from build123d import *

# Parameters (mm, degrees)
SKETCH1_R                  = 15
BOSS_EXTRUDE1_DEPTH        = 10
SKETCH2_R                  = 10.1
CUT_EXTRUDE1_DEPTH         = 20
SKETCH3_R                  = 15
BOSS_EXTRUDE2_DEPTH        = 10
SKETCH5_R                  = 10
CUT_EXTRUDE3_DEPTH         = 8
SKETCH8_W                  = 0.75
SKETCH8_H                  = 0.75
CUT_EXTRUDE5_DEPTH         = 2
FILL_START                 = -1.125
FILL_PATTERN2_OUTLINE_W    = 0.75
FILL_PATTERN2_OUTLINE_H    = 2
FILL_PATTERN2_DEPTH        = 0.75
FILL_START_2               = 0.375
FILL_PATTERN2_2_OUTLINE_W  = 0.75
FILL_PATTERN2_2_OUTLINE_H  = 2
FILL_PATTERN2_2_DEPTH      = 0.75
FILL_START_3               = -3.375
FILL_PATTERN2_3_OUTLINE_W  = 0.75
FILL_PATTERN2_3_OUTLINE_H  = 2
FILL_PATTERN2_3_DEPTH      = 0.75
FILL_START_4               = -1.875
FILL_PATTERN2_4_OUTLINE_W  = 0.75
FILL_PATTERN2_4_OUTLINE_H  = 2
FILL_PATTERN2_4_DEPTH      = 0.75
FILL_START_5               = 1.125
FILL_PATTERN2_5_OUTLINE_W  = 0.75
FILL_PATTERN2_5_OUTLINE_H  = 2
FILL_PATTERN2_5_DEPTH      = 0.75
FILL_START_6               = 2.625
FILL_PATTERN2_6_OUTLINE_W  = 0.75
FILL_PATTERN2_6_OUTLINE_H  = 2
FILL_PATTERN2_6_DEPTH      = 0.75
FILL_START_7               = -4.125
FILL_PATTERN2_7_OUTLINE_W  = 0.75
FILL_PATTERN2_7_OUTLINE_H  = 2
FILL_PATTERN2_7_DEPTH      = 0.75
FILL_START_8               = -2.625
FILL_PATTERN2_8_OUTLINE_W  = 0.75
FILL_PATTERN2_8_OUTLINE_H  = 2
FILL_PATTERN2_8_DEPTH      = 0.75
FILL_START_9               = -0.375
FILL_PATTERN2_9_OUTLINE_W  = 0.75
FILL_PATTERN2_9_OUTLINE_H  = 2
FILL_PATTERN2_9_DEPTH      = 0.75
FILL_START_10              = 1.875
FILL_PATTERN2_10_OUTLINE_W = 0.75
FILL_PATTERN2_10_OUTLINE_H = 2
FILL_PATTERN2_10_DEPTH     = 0.75
FILL_START_11              = 3.375
FILL_PATTERN2_11_OUTLINE_W = 0.75
FILL_PATTERN2_11_OUTLINE_H = 2
FILL_PATTERN2_11_DEPTH     = 0.75
SKETCH15_W                 = 16
SKETCH15_H                 = 2.5
SKETCH16_R                 = 1.2


# Read off the part's stored shape, not the designer's step: Fill Pattern2
with BuildPart() as part:
    # Sketch1 → Boss-Extrude1 (new body)
    with BuildSketch(Plane.XY):
        Circle(SKETCH1_R)
    extrude(amount=BOSS_EXTRUDE1_DEPTH)

    # Sketch2 → Cut-Extrude1 (cut)
    with BuildSketch(Plane.XY.offset(10)):
        Circle(SKETCH2_R)
    extrude(amount=-CUT_EXTRUDE1_DEPTH, mode=Mode.SUBTRACT)

    # Sketch3 → Boss-Extrude2 (add)
    with BuildSketch(Plane.XY.offset(10)):
        Circle(SKETCH3_R)
    extrude(amount=BOSS_EXTRUDE2_DEPTH)

    # Sketch5 → Cut-Extrude3 (cut)
    with BuildSketch(Plane.XY.offset(20)):
        Circle(SKETCH5_R)
    extrude(amount=-CUT_EXTRUDE3_DEPTH, mode=Mode.SUBTRACT)

    # Sketch8 → Cut-Extrude5 (cut)
    with BuildSketch(Plane(origin=(0, 0, 10), x_dir=(-1, 0, 0), z_dir=(0, 0, -1))):
        Rectangle(SKETCH8_W, SKETCH8_H)
    extrude(amount=-CUT_EXTRUDE5_DEPTH, mode=Mode.SUBTRACT)

    # Fill Pattern2 outline → Fill Pattern2 (cut)
    with BuildSketch(Plane.YZ.offset(FILL_START)):
        with Locations((-1.299038106, 11)):
            Rectangle(FILL_PATTERN2_OUTLINE_W, FILL_PATTERN2_OUTLINE_H)
        with Locations((1.299038106, 11)):
            Rectangle(FILL_PATTERN2_OUTLINE_W, FILL_PATTERN2_OUTLINE_H)
        with Locations((-3.897114317, 11)):
            Rectangle(FILL_PATTERN2_OUTLINE_W, FILL_PATTERN2_OUTLINE_H)
        with Locations((3.897114317, 11)):
            Rectangle(FILL_PATTERN2_OUTLINE_W, FILL_PATTERN2_OUTLINE_H)
    extrude(amount=FILL_PATTERN2_DEPTH, mode=Mode.SUBTRACT)

    # Fill Pattern2 2 outline → Fill Pattern2 2 (cut)
    with BuildSketch(Plane.YZ.offset(FILL_START_2)):
        with Locations((-1.299038106, 11)):
            Rectangle(FILL_PATTERN2_2_OUTLINE_W, FILL_PATTERN2_2_OUTLINE_H)
        with Locations((1.299038106, 11)):
            Rectangle(FILL_PATTERN2_2_OUTLINE_W, FILL_PATTERN2_2_OUTLINE_H)
        with Locations((-3.897114317, 11)):
            Rectangle(FILL_PATTERN2_2_OUTLINE_W, FILL_PATTERN2_2_OUTLINE_H)
        with Locations((3.897114317, 11)):
            Rectangle(FILL_PATTERN2_2_OUTLINE_W, FILL_PATTERN2_2_OUTLINE_H)
    extrude(amount=FILL_PATTERN2_2_DEPTH, mode=Mode.SUBTRACT)

    # Fill Pattern2 3 outline → Fill Pattern2 3 (cut)
    with BuildSketch(Plane.YZ.offset(FILL_START_3)):
        with Locations((0, 11)):
            Rectangle(FILL_PATTERN2_3_OUTLINE_W, FILL_PATTERN2_3_OUTLINE_H)
        with Locations((-2.598076211, 11)):
            Rectangle(FILL_PATTERN2_3_OUTLINE_W, FILL_PATTERN2_3_OUTLINE_H)
        with Locations((2.598076211, 11)):
            Rectangle(FILL_PATTERN2_3_OUTLINE_W, FILL_PATTERN2_3_OUTLINE_H)
    extrude(amount=FILL_PATTERN2_3_DEPTH, mode=Mode.SUBTRACT)

    # Fill Pattern2 4 outline → Fill Pattern2 4 (cut)
    with BuildSketch(Plane.YZ.offset(FILL_START_4)):
        with Locations((0, 11)):
            Rectangle(FILL_PATTERN2_4_OUTLINE_W, FILL_PATTERN2_4_OUTLINE_H)
        with Locations((-2.598076211, 11)):
            Rectangle(FILL_PATTERN2_4_OUTLINE_W, FILL_PATTERN2_4_OUTLINE_H)
        with Locations((2.598076211, 11)):
            Rectangle(FILL_PATTERN2_4_OUTLINE_W, FILL_PATTERN2_4_OUTLINE_H)
    extrude(amount=FILL_PATTERN2_4_DEPTH, mode=Mode.SUBTRACT)

    # Fill Pattern2 5 outline → Fill Pattern2 5 (cut)
    with BuildSketch(Plane.YZ.offset(FILL_START_5)):
        with Locations((0, 11)):
            Rectangle(FILL_PATTERN2_5_OUTLINE_W, FILL_PATTERN2_5_OUTLINE_H)
        with Locations((-2.598076211, 11)):
            Rectangle(FILL_PATTERN2_5_OUTLINE_W, FILL_PATTERN2_5_OUTLINE_H)
        with Locations((2.598076211, 11)):
            Rectangle(FILL_PATTERN2_5_OUTLINE_W, FILL_PATTERN2_5_OUTLINE_H)
    extrude(amount=FILL_PATTERN2_5_DEPTH, mode=Mode.SUBTRACT)

    # Fill Pattern2 6 outline → Fill Pattern2 6 (cut)
    with BuildSketch(Plane.YZ.offset(FILL_START_6)):
        with Locations((0, 11)):
            Rectangle(FILL_PATTERN2_6_OUTLINE_W, FILL_PATTERN2_6_OUTLINE_H)
        with Locations((-2.598076211, 11)):
            Rectangle(FILL_PATTERN2_6_OUTLINE_W, FILL_PATTERN2_6_OUTLINE_H)
        with Locations((2.598076211, 11)):
            Rectangle(FILL_PATTERN2_6_OUTLINE_W, FILL_PATTERN2_6_OUTLINE_H)
    extrude(amount=FILL_PATTERN2_6_DEPTH, mode=Mode.SUBTRACT)

    # Fill Pattern2 7 outline → Fill Pattern2 7 (cut)
    with BuildSketch(Plane.YZ.offset(FILL_START_7)):
        with Locations((-1.299038106, 11)):
            Rectangle(FILL_PATTERN2_7_OUTLINE_W, FILL_PATTERN2_7_OUTLINE_H)
        with Locations((1.299038106, 11)):
            Rectangle(FILL_PATTERN2_7_OUTLINE_W, FILL_PATTERN2_7_OUTLINE_H)
    extrude(amount=FILL_PATTERN2_7_DEPTH, mode=Mode.SUBTRACT)

    # Fill Pattern2 8 outline → Fill Pattern2 8 (cut)
    with BuildSketch(Plane.YZ.offset(FILL_START_8)):
        with Locations((-1.299038106, 11)):
            Rectangle(FILL_PATTERN2_8_OUTLINE_W, FILL_PATTERN2_8_OUTLINE_H)
        with Locations((1.299038106, 11)):
            Rectangle(FILL_PATTERN2_8_OUTLINE_W, FILL_PATTERN2_8_OUTLINE_H)
    extrude(amount=FILL_PATTERN2_8_DEPTH, mode=Mode.SUBTRACT)

    # Fill Pattern2 9 outline → Fill Pattern2 9 (cut)
    with BuildSketch(Plane.YZ.offset(FILL_START_9)):
        with Locations((-2.598076211, 11)):
            Rectangle(FILL_PATTERN2_9_OUTLINE_W, FILL_PATTERN2_9_OUTLINE_H)
        with Locations((2.598076211, 11)):
            Rectangle(FILL_PATTERN2_9_OUTLINE_W, FILL_PATTERN2_9_OUTLINE_H)
    extrude(amount=FILL_PATTERN2_9_DEPTH, mode=Mode.SUBTRACT)

    # Fill Pattern2 10 outline → Fill Pattern2 10 (cut)
    with BuildSketch(Plane.YZ.offset(FILL_START_10)):
        with Locations((-1.299038106, 11)):
            Rectangle(FILL_PATTERN2_10_OUTLINE_W, FILL_PATTERN2_10_OUTLINE_H)
        with Locations((1.299038106, 11)):
            Rectangle(FILL_PATTERN2_10_OUTLINE_W, FILL_PATTERN2_10_OUTLINE_H)
    extrude(amount=FILL_PATTERN2_10_DEPTH, mode=Mode.SUBTRACT)

    # Fill Pattern2 11 outline → Fill Pattern2 11 (cut)
    with BuildSketch(Plane.YZ.offset(FILL_START_11)):
        with Locations((-1.299038106, 11)):
            Rectangle(FILL_PATTERN2_11_OUTLINE_W, FILL_PATTERN2_11_OUTLINE_H)
        with Locations((1.299038106, 11)):
            Rectangle(FILL_PATTERN2_11_OUTLINE_W, FILL_PATTERN2_11_OUTLINE_H)
    extrude(amount=FILL_PATTERN2_11_DEPTH, mode=Mode.SUBTRACT)

    # Sketch15 → Revolve2 (revolve)
    with BuildSketch(Plane(origin=(0, 0, 0), x_dir=(0, 0, -1), z_dir=(1, 0, 0)), mode=Mode.PRIVATE) as revolve2_sk:
        with Locations((-20, -8.75)):
            Rectangle(SKETCH15_W, SKETCH15_H)
    revolve(revolve2_sk.sketch.rotate(Axis((0, 0, 20), (0, 0, -1)), 270), axis=Axis((0, 0, 20), (0, 0, -1)))

    # Sketch16 → Cut-Revolve2 (revolve, cut)
    with BuildSketch(Plane(origin=(0, 0, 0), x_dir=(0, 0, -1), z_dir=(1, 0, 0)), mode=Mode.PRIVATE) as cut_revolve2_sk:
        with Locations((-23, 10)):
            Circle(SKETCH16_R)
    revolve(cut_revolve2_sk.sketch.rotate(Axis((0, 0, 20), (0, 0, -1)), 90), axis=Axis((0, 0, 20), (0, 0, -1)), mode=Mode.SUBTRACT)


solid = part.part
Geometry check sheet. Reference: the model listing, model coordinates, mm. A direction names the side the tool comes from. Round coordinates to 2 decimals unless told otherwise and drop trailing zeros. Loops run counter-clockwise (first coordinate to the right, second up) from the corner with the lowest first, then second, coordinate; pieces in that order, holes last. Notation, with made-up numbers: (4.5, -14) -> (10.5, -14) arc R26 cw to (10.5, 22) -> close; hole circle Ø3 at (-8.5, 63.5). An arc over 180 degrees is marked (long way). Answer as a JSON object with one key per item and string values. Group by question number.
Item 1: Cross-section at A-A, the plane z = 26.25. Record the cut outline in (x, y), plus the area to 3 significant figures.
Item 2: Cross-section at C-C, the plane z = 4. Record the cut outline in (x, y), plus the area to 3 significant figures.
Item 3: Set-up check for faces 4 (the face through (-7.493, -0.33, 19.888)), 5 (the face through (0, -2, 10)), 6 (the face through (3, -10, 0)): record each of +Z, -Z, +X, -X, +Y, -Y from which the full face is reachable in a straight line by a thin tool's end or side.
Item 4: Release check for a two-part mould opening along X. For faces 1 (the face through (4, -7, 28)), 2 (the face through (9.634, 3.034, 5.07)), 3 (the face through (-2.17, 9.76, 20.89)) record: pulls with the +X half, pulls with the -X half, needs draft (parallel to the pull), parting line crosses it, or undercut.
Item 5: Cross-section at B-B, the plane x = -13. Record the cut outline in (y, z), plus the area to 3 significant figures.
Item 6: Thickness scan on line 1 along Y through (x, z) = (0, 7); line 2 along Z through (x, y) = (-5.75, -8); line 3 along Y through (x, z) = (0, 16.5). Record the ranges inside material, lowest first.
Item 7: Depth check by flat-ended pin: pin 1 Ø2 at (y, z) = (-3, 6) entering from +X; pin 2 Ø13.5 at (x, y) = (0, 0) entering from -Z; pin 3 Ø1.5 at (y, z) = (-5.5, 5) entering from +X. Enter the tip coordinate at first touch or a pass-through.
Determined:
{
 "1": {"outline": "circle Ø20 at (0, 0); hole circle Ø15 at (0, 0)", "area": "137 mm²"},
 "2": {"outline": "circle Ø30 at (0, 0); hole circle Ø20.2 at (0, 0)", "area": "386 mm²"},
 "3": {"face 4": "+Z", "face 5": "-Z", "face 6": "-Z, +X, -X, +Y, -Y"},
 "4": {"face 1": "needs draft", "face 2": "undercut", "face 3": "parting line crosses it"},
 "5": {"outline": "(-7.48, 0) -> (7.48, 0) -> (7.48, 20) -> (-7.48, 20) -> close", "area": "299 mm²"},
 "6": {"line 1": "y = -15 to -10.1, 10.1 to 15", "line 2": "z = 10 to 21.81, 24.19 to 28", "line 3": "y = -15 to -7.5, 7.5 to 15"},
 "7": {"pin 1": "stops at x = 14.87", "pin 2": "stops at z = 10", "pin 3": "stops at x = 14.23"}
}
